```python
from build123d import *

# Parameters (mm, degrees)
F0_W     = 56.8
F0_H     = 49.16
F1_DEPTH = 4.83
F2_SIZE  = 1
F4_DEPTH = 5.08
F5_R     = 1.95
F6_DEPTH = 25
F5_W     = 14.2
F5_H     = 13.64
F7_DEPTH = 5.06


with BuildPart() as f1:
    # F0 (on Front) → F1 (new body)
    with BuildSketch(Plane.XZ):
        Rectangle(F0_W, F0_H)
    extrude(amount=F1_DEPTH)

    # F2
    f2_edges = [f1.edges().sort_by_distance(p)[0] for p in [
        (28.4, -4.83, 0),
        (0, -4.83, 24.58),
        (-28.4, -4.83, 0),
        (0, -4.83, -24.58),
    ]]
    chamfer(f2_edges, length=F2_SIZE)

    # F3 (on face) → F4 (join)
    with BuildSketch(Plane(origin=(0, 0, 0), x_dir=(-1, 0, 0), z_dir=(0, 1, 0))):
        Polygon((23.75, 17.29), (17.64, 17.29), (17.64, 14.84), (21.3, 14.84), (21.3, 11.18), (23.75, 11.18), align=None)
        Polygon((-18.37, -10.69), (-20.82, -10.69), (-20.82, -16.8), (-14.71, -16.8), (-14.71, -14.35), (-18.37, -14.35), align=None)
        Polygon((23.75, -16.8), (23.75, -10.69), (21.3, -10.69), (21.3, -14.35), (17.64, -14.35), (17.64, -16.8), align=None)
        Polygon((-14.71, 17.29), (-20.82, 17.29), (-20.82, 11.18), (-18.37, 11.18), (-18.37, 14.84), (-14.71, 14.84), align=None)
    extrude(amount=F4_DEPTH)

    # F5 (on face) → F6 (cut)
    with BuildSketch(Plane(origin=(0, 0, 0), x_dir=(-1, 0, 0), z_dir=(0, 1, 0))):
        with Locations((11.9, 6.82)):
            Circle(F5_R)
        with Locations((11.9, -6.82)):
            Circle(F5_R)
    extrude(amount=-F6_DEPTH, mode=Mode.SUBTRACT)

    # F5 (on face) → F7 (join)
    with BuildSketch(Plane(origin=(0, 0, 0), x_dir=(-1, 0, 0), z_dir=(0, 1, 0))):
        Polygon((19, 0.28), (19, 13.92), (4.8, 13.92), (4.8, 0.28), (4.8, -0.28), (19, -0.28), align=None)
        Polygon((13.957583, 10.278321), (15.923786, 6.767241), (13.866202, 3.30892), (9.842417, 3.361679), (7.876214, 6.872759), (9.933798, 10.33108), align=None, mode=Mode.SUBTRACT)
        with Locations((11.9, -7.1)):
            Rectangle(F5_W, F5_H)
        Polygon((9.933798, -10.33108), (7.876214, -6.872759), (9.842417, -3.361679), (13.866202, -3.30892), (15.923786, -6.767241), (13.957583, -10.278321), align=None, mode=Mode.SUBTRACT)
    extrude(amount=F7_DEPTH)


solid = f1.part
```
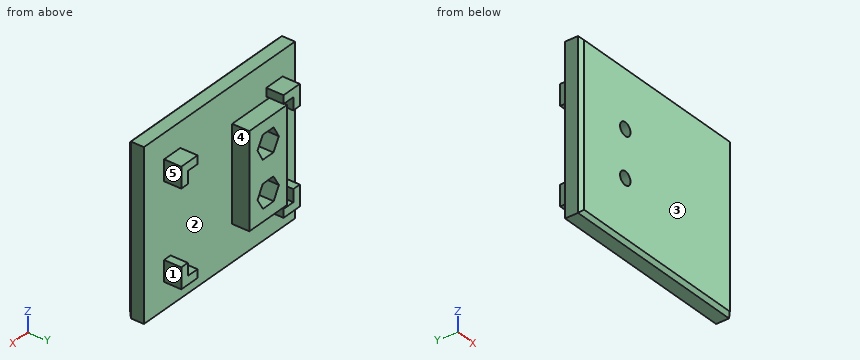
Can you work these out from the model? Positions are in its coordinate system, mm. Face numbers are marked on the shaded views. A direction names the side the tool comes from. Round coordinates to 2 decimals unless told otherwise and drop trailing zeros. Loops run counter-clockwise (first coordinate to the right, second up) from the corner with the lowest first, then second, coordinate; pieces in that order, holes last. Notation, with made-up numbers: (43, 40.25) -> (82, 40.25) arc R19 ccw to (82, 62.25) -> close; hole circle Ø8 at (52.5, 70.25). An arc over 180 degrees is marked (long way). Answer in a Markdown table with one row per item.
Item 1: If I drill on probe 1 along Z at (x, y) = (-11.9, -2); probe 2 along Z at (x, y) = (19, 0.5); probe 3 along Y at (x, z) = (-22.5, 10), over which ranges is the centre line in solid material (lowest first)?
Answer block:
| item | result |
|---|---|
| probe 1 | -24.58 to -8.77, -4.87 to 4.87, 8.77 to 24.58 |
| probe 2 | -16.8 to -10.69, 11.18 to 17.29 |
| probe 3 | -4.83 to 0 |
Item 2: On a 3-axis mill with a long thin cutter (end or side, diameter ignored), from which of +Z, -Z, +X, -X, +Y, -Y can I reach the whole of each face in a straight line? I mean the marked faces 3, 4 and 5. Say none if no direction works.
Answer block:
| item | result |
|---|---|
| face 3 | +Z, -Z, +X, -X, -Y |
| face 4 | +Z, -Z, +Y |
| face 5 | +Z, -Z, +X, +Y |
Item 3: We'd pull the mould along X, two halves only. Please class the marked faces 1 and 2: released by +X, released by -X, zero draft, split by the parting line, or undercut.
Answer block:
| item | result |
|---|---|
| face 1 | released by +X |
| face 2 | undercut |
Item 4: Suppose I cut it at D-D, the plane z = -19. List the corners of the cut face in (x, y) for me.
Answer block:
| item | result |
|---|---|
| outline | (-28.4, -3.83) -> (-27.4, -4.83) -> (27.4, -4.83) -> (28.4, -3.83) -> (28.4, 0) -> (-28.4, 0) -> close |
Item 5: Will these pins go through, and if not, where does the flat tip stop? P1, Ø2, axis at x = -11, z = -8, coming from the +Y side; P2, Ø1.8, axis at x = 17, y = 3.5, coming from the +Z side; P3, Ø1.5, axis at y = 3.5, z = -2.5, coming from the +X side; P4, Ø5.5, axis at x = -19.5, y = 1.5, coming from the +Z side.
Answer block:
| item | result |
|---|---|
| P1 | y = 0 |
| P2 | z = 17.29 |
| P3 | x = -4.8 |
| P4 | z = 24.58 |
Item 6: Suppose I cut it at A-A, the plane x = -22.5. List the corners of the cut face in (y, z) for me.
Answer block:
| item | result |
|---|---|
| outline | (-4.83, -23.58) -> (-3.83, -24.58) -> (0, -24.58) -> (0, -16.8) -> (5.08, -16.8) -> (5.08, -10.69) -> (0, -10.69) -> (0, 11.18) -> (5.08, 11.18) -> (5.08, 17.29) -> (0, 17.29) -> (0, 24.58) -> (-3.83, 24.58) -> (-4.83, 23.58) -> close |
Item 7: Suppose I cut it at C-C, the plane x = -11.9. List the corners of the cut face in (y, z) for me.
Answer block:
| item | result |
|---|---|
| outline | (-4.83, -23.58) -> (-3.83, -24.58) -> (0, -24.58) -> (0, -13.92) -> (5.06, -13.92) -> (5.06, -10.31) -> (0, -10.31) -> (0, -8.77) -> (-4.83, -8.77) -> close; (-4.83, -4.87) -> (0, -4.87) -> (0, -3.33) -> (5.06, -3.33) -> (5.06, 3.33) -> (0, 3.33) -> (0, 4.87) -> (-4.83, 4.87) -> close; (-4.83, 8.77) -> (0, 8.77) -> (0, 10.31) -> (5.06, 10.31) -> (5.06, 13.92) -> (0, 13.92) -> (0, 24.58) -> (-3.83, 24.58) -> (-4.83, 23.58) -> close |
Item 8: Suppose I cut it at B-B, the plane z = 7.5. List the corners of the cut face in (x, y) for me, plus the area to 3 significant figures.
Answer block:
| item | result |
|---|---|
| outline | (-28.4, -3.83) -> (-27.4, -4.83) -> (-13.73, -4.83) -> (-13.73, 0) -> (-15.51, 0) -> (-15.51, 5.06) -> (-19, 5.06) -> (-19, 0) -> (-28.4, 0) -> close; (-10.07, -4.83) -> (27.4, -4.83) -> (28.4, -3.83) -> (28.4, 0) -> (-4.8, 0) -> (-4.8, 5.06) -> (-8.25, 5.06) -> (-8.25, 0) -> (-10.07, 0) -> close |
| area | 291 mm² |
